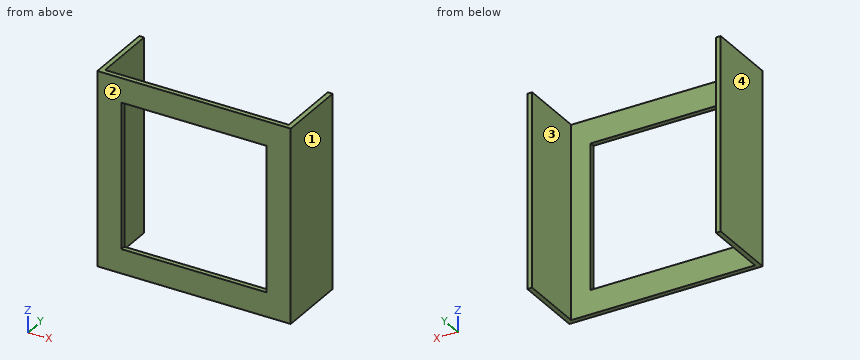
```python
from build123d import *

# Parameters (mm, degrees)
F0_W     = 80
F0_H     = 80
F0_W_2   = 60
F0_H_2   = 60
F1_DEPTH = 2
F2_W     = 2
F2_H     = 80
F3_DEPTH = 27


with BuildPart() as f1:
    # F0 (on Front) → F1 (new body)
    with BuildSketch(Plane.XZ):
        Rectangle(F0_W, F0_H)
        Rectangle(F0_W_2, F0_H_2, mode=Mode.SUBTRACT)
    extrude(amount=F1_DEPTH)

    # F2 (on face) → F3 (join)
    with BuildSketch(Plane(origin=(0, 0, 0), x_dir=(-1, 0, 0), z_dir=(0, 1, 0))):
        with Locations((-39, 0)):
            Rectangle(F2_W, F2_H)
        with Locations((39, 0)):
            Rectangle(F2_W, F2_H)
    extrude(amount=F3_DEPTH)


solid = f1.part
```
The listing builds one solid part. Answer for the finished solid, in the listing's coordinates (mm). Face numbers are marked on the shaded views. Coordinates: 2 decimals unless noted, no trailing zeros. Loops run counter-clockwise (first coordinate to the right, second up) from the corner with the lowest first, then second, coordinate; pieces in that order, holes last. Notation, with made-up numbers: (40.5, 32) - (68.5, 32) arc R16 cw to (68.5, 62) - close; hole circle Ø1 at (-9.75, 50.25). An arc over 180 degrees is marked (long way). Use a Markdown table: item, result. Add a question column.
1) The part is cut by section C-C, the plane z = 9. Give the vertices of the cut face in (x, y).
2) The part is cut by section B-B, the plane x = 9.5. Give the vertices of the cut face in (y, z), and give its area (3 significant figures).
3) The part is cut by section A-A, the plane y = 12. Give the vertices of the cut face in (x, z).
4) The part is cut by section D-D, the plane z = -34.5. Give the vertices of the cut face in (x, y), and give its area (3 significant figures).
5) The mould has two halves that part along X. Classify the marked faces 1, 2, 3 and 4: released by +X, released by -X, zero draft, split by the parting line, or undercut.
6) Find the intervals of material crossed by line 1 (X direction, y = 9.75, z = -6); line 2 (Y direction, x = -11.5, z = -33.5), in increasing order.
Here are the results:
| question | item | result |
|---|---|---|
| 1 | outline | (-40, -2) - (-30, -2) - (-30, 0) - (-38, 0) - (-38, 27) - (-40, 27) - close; (30, -2) - (40, -2) - (40, 27) - (38, 27) - (38, 0) - (30, 0) - close |
| 2 | outline | (-2, -40) - (0, -40) - (0, -30) - (-2, -30) - close; (-2, 30) - (0, 30) - (0, 40) - (-2, 40) - close |
| 2 | area | 40.0 mm^2 |
| 3 | outline | (-40, -40) - (-38, -40) - (-38, 40) - (-40, 40) - close; (38, -40) - (40, -40) - (40, 40) - (38, 40) - close |
| 4 | outline | (-40, -2) - (40, -2) - (40, 27) - (38, 27) - (38, 0) - (-38, 0) - (-38, 27) - (-40, 27) - close |
| 4 | area | 268 mm^2 |
| 5 | face 1 | released by +X |
| 5 | face 2 | zero draft |
| 5 | face 3 | undercut |
| 5 | face 4 | released by -X |
| 6 | line 1 | x = -40 to -38, 38 to 40 |
| 6 | line 2 | y = -2 to 0 |
